Check sheet for the modelled part. Datum: model origin and axes. Units: mm. A direction names the side the tool comes from. Round coordinates to 2 decimals unless told otherwise and drop trailing zeros. Write each loop counter-clockwise with the first axis right and the second up, starting at its lowest first coordinate (ties: lowest second). Pieces come first, ordered by that corner, then holes.
Item 1: Material ranges on line 1 along X through (y, z) = (0.5, 225) (1 decimal); line 2 along Z through (x, y) = (0, 10.25), recorded low to high.
Item 2: Section check A-A, the plane z = 94. Record the cut outline in (x, y) (1 decimal), plus the area to 3 significant figures.
Item 3: Set-up check for faces 4 (the flat face through (0, 9.525, 247)), 5 (the flat face through (10, 0, 501.65)): record each of +Z, -Z, +X, -X, +Y, -Y from which the full face is reachable in a straight line by a thin tool's end or side.
Item 4: Release check for a two-part mould opening along Y. For faces 1 (the flat face through (10.986, 0, 247)), 2 (the flat face through (-9.525, 0, 247)), 3 (the flat face through (0, 10.986, 247)) record: pulls with the +Y half, pulls with the -Y half, needs draft (parallel to the pull), parting line crosses it, or undercut.
from build123d import *

# Parameters (mm, degrees)
SKETCH4_W                  = 21.971
SKETCH4_H                  = 21.971
SKETCH4_W_2                = 19.05
SKETCH4_H_2                = 19.05
BOSS_EXTRUDE2_DEPTH        = 501.65
FILLET1_R                  = 2.54
F_10_CLEARANCE_HOLE1_D     = 5.1054
F_10_CLEARANCE_HOLE1_DEPTH = 16.51
F_10_CLEARANCE_HOLE1_TIP   = 1.533816902
F_10_CLEARANCE_HOLE2_D     = 5.1054


with BuildPart() as part:
    # Sketch4 → Boss-Extrude2 (new body)
    with BuildSketch(Plane.XY):
        Rectangle(SKETCH4_W, SKETCH4_H)
        Rectangle(SKETCH4_W_2, SKETCH4_H_2, mode=Mode.SUBTRACT)
    extrude(amount=BOSS_EXTRUDE2_DEPTH)

    # Fillet1
    fillet1_edges = [part.edges().sort_by_distance(p)[0] for p in [
        (-10.9855, 10.9855, 250.825),
        (10.9855, 10.9855, 250.825),
        (10.9855, -10.9855, 250.825),
        (-10.9855, -10.9855, 250.825),
    ]]
    fillet(fillet1_edges, radius=FILLET1_R)

    # #10 Clearance Hole1
    with Locations(Plane(origin=(0, 10.9855, 0), x_dir=(1, 0, 0), z_dir=(0, 1, 0))):
        with Locations((0, -12.7)):
            Hole(F_10_CLEARANCE_HOLE1_D / 2, depth=F_10_CLEARANCE_HOLE1_DEPTH)
            with Locations((0, 0, -(F_10_CLEARANCE_HOLE1_DEPTH + F_10_CLEARANCE_HOLE1_TIP / 2))):  # 118° drill point
                Cone(0, F_10_CLEARANCE_HOLE1_D / 2, F_10_CLEARANCE_HOLE1_TIP, mode=Mode.SUBTRACT)

    # #10 Clearance Hole2 (through all)
    with Locations(Plane(origin=(10.9855, 0, 0), x_dir=(0, 0, -1), z_dir=(1, 0, 0))):
        with Locations((-488.95, 0)):
            Hole(F_10_CLEARANCE_HOLE2_D / 2)


solid = part.part
Values found:
1. line 1: x = -11 to -9.5, 9.5 to 11
1. line 2: z = 0 to 10.15, 15.25 to 501.65
2. outline: (-11, -8.4) arc R2.5 ccw to (-8.4, -11) - (8.4, -11) arc R2.5 ccw to (11, -8.4) - (11, 8.4) arc R2.5 ccw to (8.4, 11) - (-8.4, 11) arc R2.5 ccw to (-11, 8.4) - close; hole (-9.5, -9.5) - (9.5, -9.5) - (9.5, 9.5) - (-9.5, 9.5) - close
2. area: 114 mm2
3. face 4: +Z, -Z
3. face 5: +Z, +X, -X, +Y, -Y
4. face 1: needs draft
4. face 2: undercut
4. face 3: pulls with the +Y half
